Check sheet for the modelled part. Datum: model origin and axes. Units: mm. Face numbers are marked on the shaded views. A direction names the side the tool comes from. Give positions to 0.01 mm unless a question says otherwise; leave off trailing zeros. Loops run counter-clockwise (first coordinate to the right, second up) from the corner with the lowest first, then second, coordinate; pieces in that order, holes last. Notation, with made-up numbers: (42, 67) -> (85, 67) arc R26 cw to (85, 99) -> close; hole circle Ø7 at (65.5, -4.75). An arc over 180 degrees is marked (long way). Answer as CSV lines item,"result". Start each with the question number.
(1) Gauge pin test, flat ends, axial feed: pin 1 Ø14.5 at (y, z) = (-20, -46.5) entering from +X; pin 2 Ø8.5 at (y, z) = (-21, -44) entering from -X; pin 3 Ø1.1 at (x, y) = (-0.5, -4) entering from +Z; pin 4 Ø12 at (x, y) = (-11.5, -43) entering from +Z. Record the tip position at first contact, or that the pin passes through.
(2) Section check D-D on y = -25. Enter the section's corners in (x, z).
(3) Section check A-A on x = -3. Enter the section's corners in (y, z), plus the area to 3 significant figures.
(4) Section check B-B on y = -18. Enter the section's corners in (x, z), plus the area to 3 significant figures.
(5) Material ranges on line 1 (Y direction, x = 26, z = -52); line 2 (X direction, y = -21, z = -49); line 3 (Z direction, x = 1, y = -8.5), recorded low to high. Write a range as from..to.
(6) Section check C-C on z = -44.5. Enter the section's corners in (x, y), plus the area to 3 significant figures.
(7) Access from +Z, -Z, +X, -X, +Y, -Y to the whole of each face (thin tool, end or side, straight path). Record for the marked faces 1, 2 and 3.
from build123d import *

# Parameters (mm, degrees)
PAD002_DEPTH    = 1.1
PAD003_DEPTH    = 1
CHAMFER001_SIZE = 1


with BuildPart() as part:
    # Sketch008 → Pad002 (new body, symmetric)
    with BuildSketch(Plane.YZ):
        Polygon((-48, -68.754484), (-6, -44.754484), (-6, -44.875355), (0, -44.875355), (0, -73.754484), (-48, -73.754484), align=None)
    extrude(amount=PAD002_DEPTH, both=True)

    # Sketch009 → Pad003 (join)
    with BuildSketch(Plane(origin=(0, -5, 0), x_dir=(0, 0, -1), z_dir=(0, -1, 0))):
        Polygon((54, 5), (68, 44), (73, 44), (73, -44), (68, -44), (54, -5), align=None)
    extrude(amount=PAD003_DEPTH)

    # Chamfer001
    chamfer001_edges = [part.edges().sort_by_distance(p)[0] for p in [
        (-1.1, -27, -56.754484),
        (1.1, -27, -56.754484),
    ]]
    chamfer(chamfer001_edges, length=CHAMFER001_SIZE)


with BuildPart() as part_1:
    # Body001 placement: moved
    add(part.part.moved(Location((0, 0, 19))))


solid = part_1.part
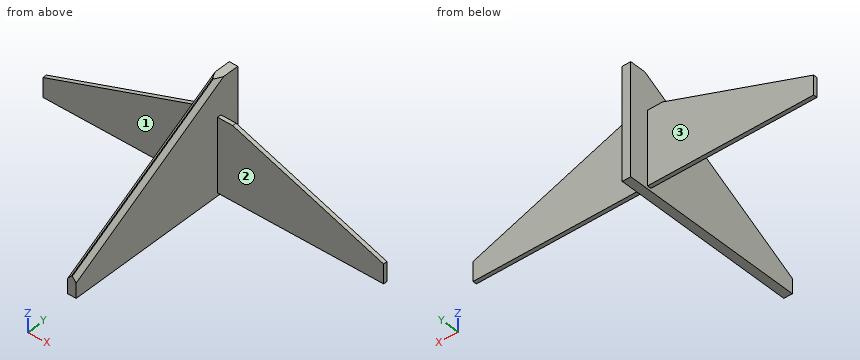
Working result:
1,pin 1,"stops at x = 1.1"
1,pin 2,"stops at x = -1.1"
1,pin 3,"stops at z = -25.88"
1,pin 4,"passes through"
2,outline,"(-1.1, -54.75) -> (1.1, -54.75) -> (1.1, -37.76) -> (0.1, -36.61) -> (-0.1, -36.61) -> (-1.1, -37.76) -> close"
3,outline,"(-6, -54) -> (-5, -54) -> (-5, -35) -> (-6, -35) -> close"
3,area,"19.0 mm^2"
4,outline,"(-1.1, -54.75) -> (1.1, -54.75) -> (1.1, -33.76) -> (0.1, -32.61) -> (-0.1, -32.61) -> (-1.1, -33.76) -> close"
4,area,"47.6 mm^2"
5,line 1,"y = -6..-5"
5,line 2,"x = -1.1..1.1"
5,line 3,"z = -54.75..-28.22"
6,outline,"(-31.46, -6) -> (-1.1, -6) -> (-1.1, -36.79) -> (-0.1, -38.8) -> (0.1, -38.8) -> (1.1, -36.79) -> (1.1, -6) -> (31.46, -6) -> (31.46, -5) -> (1.1, -5) -> (1.1, 0) -> (-1.1, 0) -> (-1.1, -5) -> (-31.46, -5) -> close"
6,area,"144 mm^2"
7,face 1,"+Z, -Z, -X, -Y"
7,face 2,"+Z, -Z, +X, -Y"
7,face 3,"+Z, -Z, -X, +Y"
